Autodesk Fusion 360 part; units mm, degrees
sketch "Sketch1" plane through (0, 0, 0) normal (0, 1, 0) x (1, 0, 0)
  line L0 (0, 0) -> (230.6, 0)
  line L1 (230.6, 0) -> (230.6, 183)
  line L2 (230.6, 183) -> (0, 183)
  line L3 (0, 183) -> (0, 0)
  dimension "d1" = 230.6
  dimension "d2" = 183
extrude "Extrude1" add sketch "Sketch1" along normal blind 10
sketch "Sketch9" plane through (0, 0, 0) normal (-1, 0, 0) x (0, 0, 1)
  line L0 (-183, 0) -> (0, 0)
  line L1 (0, 0) -> (0, 10)
  line L2 (0, 10) -> (-183, 10)
  line L3 (-183, 10) -> (-183, 0)
  circle A0 centre (11.4881, 10.5) radius 10.5
  line L4 (11.4881, 0) -> (0, 0)
  circle A1 centre (11.4881, 10.5) radius 9
  line L5 (0, 0) -> (1, 0)
  line L6 (1, 0) -> (1, 10)
  line L7 (1, 10) -> (0, 10)
  line L8 (0, 10) -> (0, 0)
  dimension "d69" = 21
  dimension "d70" = 18
  dimension "d94" = 1
extrude "Extrude8" add sketch "Sketch9" against normal up to surface (230.6 mm away) contours L1 L4 L5 L6 L7 L8 | A0 L4 L6 | A0
sketch "Sketch10" plane through (0, 0, 0) normal (0, -1, 0) x (1, 0, 0)
  line L0 (230.6, -183) -> (230.6, 11.4881)
  line L1 (230.6, 11.4881) -> (0, 11.4881)
  line L2 (0, 11.4881) -> (0, -183)
  line L3 (230.6, 0) -> (218.6, 0)
  line L4 (218.6, 0) -> (218.6, 22)
  line L5 (218.6, 22) -> (230.6, 22)
  line L6 (230.6, 22) -> (230.6, 0)
  line L7 (203.6, 0) -> (27, 0)
  line L8 (27, 0) -> (27, 22)
  line L9 (27, 22) -> (203.6, 22)
  line L10 (203.6, 22) -> (203.6, 0)
  line L11 (0, 0) -> (12, 0)
  line L12 (12, 0) -> (12, 22)
  line L13 (12, 22) -> (0, 22)
  line L14 (0, 22) -> (0, 0)
  line L15 (0, -183) -> (230.6, -183)
  dimension "d73" = 22
  dimension "d74" = 12
  dimension "d75" = 12
  dimension "d76" = 15
  dimension "d77" = 15
extrude "Extrude9" cut sketch "Sketch10" against normal through all contours L0 L1 L3 L4 L6 | L1 L4 L5 L6 | L1 L2 L11 L12 L14 | L1 L12 L13 L14 | L1 L7 L8 L10 | L1 L8 L9 L10
sketch "Sketch11" plane through (0, 10, 0) normal (0, 1, 0) x (-1, 0, 0)
  line L0 (0, -183) -> (0, 0)
  line L1 (-1.8, -176) -> (-228.8, -176)
  line L2 (-228.8, -176) -> (-228.8, -1)
  line L3 (-228.8, -1) -> (-1.8, -1)
  line L4 (-1.8, -1) -> (-1.8, -176)
  line L5 (-115.3, -124.4699) -> (-115.3, -51.5615) construction
  line L6 (-230.6, 0) -> (-230.6, -183)
  line L7 (-230.6, -183) -> (0, -183)
  line L8 (-12, 0) -> (-12, 1)
  line L9 (-12, 1) -> (-27, 1)
  line L10 (-27, 1) -> (-27, 0)
  line L11 (-27, 0) -> (-203.6, 0)
  line L12 (-203.6, 0) -> (-203.6, 1)
  line L13 (-203.6, 1) -> (-218.6, 1)
  line L14 (-218.6, 1) -> (-218.6, 0)
  line L15 (-218.6, 0) -> (-230.6, 0)
  line L16 (0, 0) -> (-12, 0)
  dimension "d79" = 227
  dimension "d80" = 175
  dimension "d100" = 1
extrude "Extrude10" cut sketch "Sketch11" against normal blind 2 contours L1 L2 L3 L4
sketch "Sketch12" plane through (0, 8, 0) normal (0, 1, 0) x (-1, 0, 0)
  line L0 (-1.8, -1) -> (-228.8, -1)
  line L1 (-1.8, -176) -> (-1.8, -1)
  line L2 (-6.95, -6.345) -> (-223.65, -6.345)
  line L3 (-223.65, -6.345) -> (-223.65, -182.345)
  line L4 (-223.65, -182.345) -> (-6.95, -182.345)
  line L5 (-6.95, -182.345) -> (-6.95, -6.345)
  line L6 (-10.47, -167.125) -> (-220.13, -167.125)
  line L7 (-220.13, -167.125) -> (-220.13, -9.875)
  line L8 (-220.13, -9.875) -> (-10.47, -9.875)
  line L9 (-10.47, -9.875) -> (-10.47, -167.125)
  line L10 (-83.8338, -88.5) -> (-143.8338, -88.5) construction
  line L11 (-115.3, -111.7944) -> (-115.3, -61.4121) construction
  line L12 (-228.8, -1) -> (-228.8, -176)
  line L13 (-228.8, -176) -> (-1.8, -176)
  dimension "d84" = 176
  dimension "d85" = 216.7
  dimension "d86" = 209.66
  dimension "d87" = 157.25
  dimension "d88" = 3.52
  dimension "d89" = 3.53
extrude "Extrude11" cut sketch "Sketch12" against normal blind 2.6 contours L2 L3 L5 L13 | L3 L4 L5 L13 | L6 L7 L8 L9
fillet "Fillet1" radius 6 2 edges at (0, 5, -183) (230.6, 5, -183)
sketch "Sketch15" plane through (12, 0, 0) normal (-1, 0, 0) x (0, 0, 1)
  line L0 (1, 10) -> (0, 10)
  line L1 (0, 10) -> (0, 0)
  line L2 (0, 0) -> (11.4881, 0)
  arc A0 (11.4881, 0) -> (1, 10) centre (11.4881, 10.5) ccw
  circle A1 centre (11.4881, 10.5) radius 9
  circle A2 centre (11.4881, 10.5) radius 11.499
  line L3 (0, 0) -> (6.8002, 0)
extrude "Extrude14" add sketch "Sketch15" along normal blind 12 and the other way blind 218.6 contours L1 L2 A2 L3
sketch "Sketch13" plane through (0, 0, 0) normal (-1, 0, 0) x (0, 0, 1)
  line L0 (-177, 10) -> (-177, 0)
  line L1 (-177, 0) -> (6.8002, 0)
  line L2 (0, 10) -> (-177, 10)
  line L3 (-187, -4.6) -> (23, -4.6)
  line L4 (23, -4.6) -> (23, 5.4)
  line L5 (23, 5.4) -> (-187, 5.4)
  line L6 (-187, 5.4) -> (-187, -4.6)
  arc A0 (0, 10) -> (6.8002, 0) centre (11.4881, 10.5) ccw
  dimension "d95" = 4.6
  dimension "d96" = 10
  dimension "d97" = 10
  dimension "d98" = 210
extrude "Extrude12" cut sketch "Sketch13" against normal through all contours L0 L1 L5 A0 | L0 L1 L3 L4 L5 L6 A0
sketch "Sketch14" plane through (0, 5.4, 0) normal (0, -1, 0) x (1, 0, 0)
  line L0 (218.6, 18.9036) -> (218.6, 20.6663)
  line L1 (12, 18.9036) -> (27, 18.9036)
  line L2 (203.6, 20.6663) -> (203.6, 18.9036)
  line L3 (27, 18.9036) -> (27, 20.6663)
  line L4 (12, 20.6663) -> (12, 18.9036)
  line L5 (27, 20.6663) -> (12, 20.6663)
  line L6 (203.6, 18.9036) -> (218.6, 18.9036)
  line L7 (218.6, 20.6663) -> (203.6, 20.6663)
  line L8 (223.65, -8.545) -> (230.45, -8.545)
  line L9 (230.45, -8.545) -> (230.45, -168.645)
  line L10 (230.45, -168.645) -> (223.65, -168.645)
  line L11 (223.65, -168.645) -> (223.65, -8.545)
  line L12 (223.65, -182.345) -> (223.65, -6.345)
  dimension "d101" = 6.8
  dimension "d102" = 2.2
  dimension "d103" = 160.1
extrude "Extrude13" cut sketch "Sketch14" against normal blind 1.6 contours L8 L9 L10 L11 L12
The model under review builds one solid part; all positions refer to its coordinate system, in mm. A direction names the side the tool comes from. Coordinates: 2 decimals unless noted, no trailing zeros. Write each loop counter-clockwise with the first axis right and the second up, starting at its lowest first coordinate (ties: lowest second). Pieces come first, ordered by that corner, then holes. Notation, with made-up numbers: (34, 52) - (56, 52) arc R19 cw to (56, 77) - close; hole circle Ø10 at (68.25, 22.25). An arc over 180 degrees is marked (long way). Answer as a JSON object with one key per item and string values. Group by question number.
1. Add section C-C (y = 13.75). Give the boundary of the cut face in (x, z), plus the area to 3 significant figures.
2. Mouldability with a two-part tool opening along Y and no side actions: class faces 5 (the face through (117, 8, -179)), 6 (the face through (1.804, 7.732, -181.289)), 7 (the face through (19.395, 19.496, 11.762)) as pulls with the +Y half, pulls with the -Y half, needs draft (parallel to the pull), parting line crosses it, or undercut.
3. Add section A-A (x = 182). Give the boundary of the cut face in (y, z) (3 decimals).
4. To check wall thickness, follow probe 1 along X at (y, z) = (7.75, -82); probe 2 along Z at (x, y) = (25, 10.75); probe 3 along X at (y, z) = (8.25, -20.5). State the ranges of each line that lie inside material, in increasing order.
5. Add section B-B (z = -30.5). Give the boundary of the cut face in (x, y), plus the area to 3 significant figures.
6. Machinability: for faces 1 (the face through (115, 10, -180)), 2 (the face through (227, 7, -87)), 3 (the face through (116, 8, -4)), 4 (the face through (81, 5.4, -6)), which of the approach directions +Z, -Z, +X, -X, +Y, -Y give a long, thin tool a straight path to every point of the face, cutting with its end or side? Answer none if there is none.
7. Clearance check with flat-ended pins moving along their axes: pin 1 Ø1.9 at (x, z) = (83, -178.5) entering from -Y; pin 2 Ø1 at (x, y) = (112, 9) entering from +Z; pin 3 Ø1.8 at (x, y) = (226.5, 6.5) entering from +Z. State where each tip first meets the part, or that it passes through.
Findings:
{
 "1": {"outline": "(12, 1.5) - (27, 1.5) - (27, 3.1) - (12, 3.1) - close; (12, 19.88) - (27, 19.88) - (27, 21.47) - (12, 21.47) - close; (203.6, 1.5) - (218.6, 1.5) - (218.6, 3.1) - (203.6, 3.1) - close; (203.6, 19.88) - (218.6, 19.88) - (218.6, 21.47) - (203.6, 21.47) - close", "area": "95.5 mm²"},
 "2": {"face 5": "pulls with the -Y half", "face 6": "needs draft", "face 7": "undercut"},
 "3": {"outline": "(5.4, -183) - (10, -183) - (10, -176) - (8, -176) - (8, -182.345) - (5.4, -182.345) - close; (5.4, -6.345) - (8, -6.345) - (8, -1) - (10, -1) - (10, 0) arc R11.499 cw to (5.4, 1.182) - close"},
 "4": {"probe 1": "0 to 6.95, 223.65 to 230.6", "probe 2": "0.99 to 2.49, 20.48 to 21.99", "probe 3": "0 to 1.8, 228.8 to 230.6"},
 "5": {"outline": "(0, 5.4) - (6.95, 5.4) - (6.95, 8) - (1.8, 8) - (1.8, 10) - (0, 10) - close; (223.65, 7) - (230.45, 7) - (230.45, 5.4) - (230.6, 5.4) - (230.6, 10) - (228.8, 10) - (228.8, 8) - (223.65, 8) - close", "area": "32.5 mm²"},
 "6": {"face 1": "-Z, +X, -X, +Y", "face 2": "-Y", "face 3": "+Y", "face 4": "+Z, -Z, +X, -X, -Y"},
 "7": {"pin 1": "y = 8", "pin 2": "z = 0.16", "pin 3": "z = 1.09"}
}
